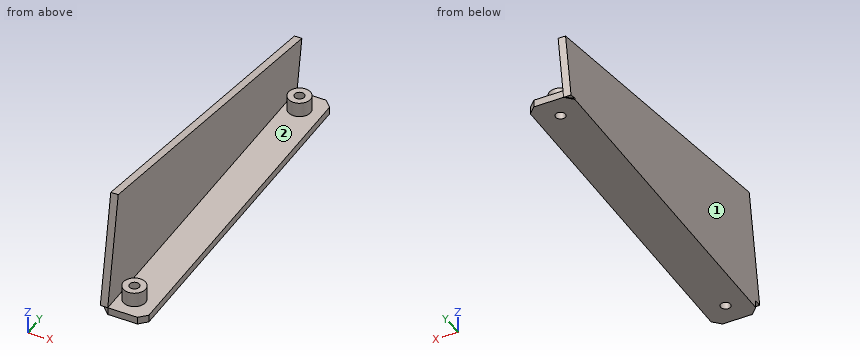
from build123d import *

# Parameters (mm, degrees)
SKETCH1_W                       = 9.525
SKETCH1_H                       = 76.2
BOSS_EXTRUDE1_DEPTH             = 1.5875
CHAMFER2_SIZE                   = 1.5875
F_97_0_0825_DIAMETER_HOLE1_D    = 2.0955
SKETCH5_R                       = 2.38125
SKETCH5_R_2                     = 1.04775
BOSS_EXTRUDE2_DEPTH             = 3.175
BOSS_EXTRUDE4_REACH             = 77.644
SKETCH7_W                       = 1.5875
SKETCH7_H                       = 75.318017262
BOSS_EXTRUDE4_DIRECTION_2_DEPTH = 12.7
BOSS_EXTRUDE5_REACH             = 79.8


with BuildPart() as part:
    # Sketch1 → Boss-Extrude1 (new body)
    with BuildSketch(Plane.XY):
        with Locations((-4.7625, 38.1)):
            Rectangle(SKETCH1_W, SKETCH1_H)
    extrude(amount=BOSS_EXTRUDE1_DEPTH)

    # Chamfer2
    chamfer2_edges = [part.edges().sort_by_distance(p)[0] for p in [
        (0, 0, 0.79375),
        (-9.525, 0, 0.79375),
        (-9.525, 76.2, 0.79375),
        (0, 76.2, 0.79375),
    ]]
    chamfer(chamfer2_edges, length=CHAMFER2_SIZE)

    # 97 _0.0825_ Diameter Hole1 (through all)
    with Locations(Plane.XY.offset(1.5875)):
        with Locations((-4.7625, 4.7625), (-4.7625, 71.4375)):
            Hole(F_97_0_0825_DIAMETER_HOLE1_D / 2)

    # Sketch5 → Boss-Extrude2 (add)
    # profile 1 of 2: a face of its own
    with BuildSketch(Plane.XY.offset(1.5875)):
        with Locations((-4.7625, 4.7625)):
            Circle(SKETCH5_R)
        with Locations((-4.7625, 4.7625)):
            Circle(SKETCH5_R_2, mode=Mode.SUBTRACT)
    # profile 2 of 2: a face of its own
    with BuildSketch(Plane.XY.offset(1.5875)):
        with Locations(Location((-4.7625, 71.4375, 0), (0, 0, 180))):
            Circle(SKETCH5_R)
        with Locations((-4.7625, 71.4375)):
            Circle(SKETCH5_R_2, mode=Mode.SUBTRACT)
    extrude(amount=BOSS_EXTRUDE2_DEPTH)

    # Boss-Extrude4: up to this face of the body (flat: up to its plane)
    boss_extrude4_end = Plane(part.part.faces().sort_by_distance((-4.7625, 38.1, 1.5875))[0])
    # Sketch7 → Boss-Extrude4 (add, up to the picked face)
    with BuildSketch(Plane(origin=(0, 2.297711148, 13.030967461), x_dir=(-1, 0, 0), z_dir=(0, -0.1736481776669307, -0.984807753012208)), mode=Mode.PRIVATE) as boss_extrude4_sk1:
        with Locations((8.73125, 37.383342149)):
            Rectangle(SKETCH7_W, SKETCH7_H)
    boss_extrude4_tool1 = split(extrude(boss_extrude4_sk1.sketch, amount=BOSS_EXTRUDE4_REACH, mode=Mode.PRIVATE), bisect_by=boss_extrude4_end, keep=Keep.BOTH, mode=Mode.PRIVATE)
    add(boss_extrude4_tool1.solids().sort_by(Axis((-8.73125, 39.113116, 6.539418), (0, -0.1736481776669307, -0.984807753012208)))[0])

    # Sketch7 → Boss-Extrude4 direction 2 (add)
    with BuildSketch(Plane(origin=(0, 2.297711148, 13.030967461), x_dir=(-1, 0, 0), z_dir=(0, -0.1736481776669307, -0.984807753012208))):
        with Locations((8.73125, 37.383342149)):
            Rectangle(SKETCH7_W, SKETCH7_H)
    extrude(amount=-BOSS_EXTRUDE4_DIRECTION_2_DEPTH)

    # Boss-Extrude5: up to this face of the body (flat: up to its plane)
    boss_extrude5_end = Plane(part.part.faces().sort_by_distance((-4.7625, 38.1, 0))[0])
    # Sketch8 → Boss-Extrude5 (add, up to the picked face)
    with BuildSketch(Plane(origin=(0, 2.297711148, 13.030967461), x_dir=(-1, 0, 0), z_dir=(0, -0.17364817766693066, -0.9848077530122081)), mode=Mode.PRIVATE) as boss_extrude5_sk1:
        Polygon((9.525, 74.993743341), (9.525, 75.04235078), (7.9375, 75.04235078), align=None)
    boss_extrude5_tool1 = split(extrude(boss_extrude5_sk1.sketch, amount=BOSS_EXTRUDE5_REACH, mode=Mode.PRIVATE), bisect_by=boss_extrude5_end, keep=Keep.BOTH, mode=Mode.PRIVATE)
    add(boss_extrude5_tool1.solids().sort_by(Axis((-8.995833, 76.184044, 0.002814), (0, -0.17364817766693066, -0.9848077530122081)))[0])


solid = part.part
Work out the finished part from the listing and answer in its coordinate system (mm). Face numbers are marked on the shaded views. Round coordinates to 2 decimals unless told otherwise and drop trailing zeros. Write each loop counter-clockwise with the first axis right and the second up, starting at its lowest first coordinate (ties: lowest second). Pieces come first, ordered by that corner, then holes. Notation, with made-up numbers: (78.5, 87.5) - (100.5, 87.5) arc R28 ccw to (100.5, 105.5) - close; hole circle Ø1 at (-13.75, -2). An arc over 180 degrees is marked (long way). Answer in a Markdown table with one row per item. Add a question column.
1. Given pin 1 (2 mm diameter, centred on x = -1, y = 21, fed in from +Z); pin 2 (4 mm diameter, centred on x = -4, y = 70.5, fed in from +Z); pin 3 (2 mm diameter, centred on x = -8, z = 12, fed in from -Y), each flat-ended and moving along its own axis, determine where each tip first touches the part or whether it passes through.
2. Find the intervals of material crossed by line 1 along X through (y, z) = (38.5, 4.5) (1 decimal); line 2 along Z through (x, y) = (-7.5, 74); line 3 along Y through (x, z) = (-3.25, 2.75), in increasing order. Write a range as from..to.
3. The mould has two halves that part along Y. Classify the marked faces 1 and 2: +Y half, -Y half, draft (parallel to the pull), parting line (faces both ways), or undercut.
4. A cutting plane is placed at B-B, the plane y = 55.5. Determine the outline of the cut face in (x, z) (1 decimal), and give its area (3 significant figures).
5. A cutting plane is placed at A-A, the plane x = -4.5. Determine the outline of the cut face in (y, z).
6. A cutting plane is placed at D-D, the plane y = 8. Determine the outline of the cut face in (x, z) (1 decimal), and give its area (3 significant figures).
7. A cutting plane is placed at C-C, the plane z = 22. Determine the outline of the cut face in (x, y) (1 decimal), and give its area (3 significant figures).
Worked out:
| question | item | result |
|---|---|---|
| 1 | pin 1 | z = 1.59 |
| 1 | pin 2 | z = 4.76 |
| 1 | pin 3 | y = 1.66 |
| 2 | line 1 | -9.5..-7.9 |
| 2 | line 2 | 0..1.59 |
| 2 | line 3 | 2.92..6.6, 69.6..73.28 |
| 3 | face 1 | draft |
| 3 | face 2 | undercut |
| 4 | outline | (-9.5, 0) - (0, 0) - (0, 1.6) - (-7.9, 1.6) - (-7.9, 16.5) - (-9.5, 16.5) - close |
| 4 | area | 38.9 mm^2 |
| 5 | outline | (0, 0) - (3.75, 0) - (3.75, 4.76) - (2.4, 4.76) - (2.4, 1.59) - (0, 1.59) - close; (5.78, 0) - (70.42, 0) - (70.42, 4.76) - (69.07, 4.76) - (69.07, 1.59) - (7.13, 1.59) - (7.13, 4.76) - (5.78, 4.76) - close; (72.45, 0) - (76.2, 0) - (76.2, 1.59) - (73.8, 1.59) - (73.8, 4.76) - (72.45, 4.76) - close |
| 6 | outline | (-9.5, 0) - (0, 0) - (0, 1.6) - (-7.9, 1.6) - (-7.9, 24.9) - (-9.5, 24.9) - close |
| 6 | area | 52.2 mm^2 |
| 7 | outline | (-9.5, 3.6) - (-7.9, 3.6) - (-7.9, 24.6) - (-9.5, 24.6) - close |
| 7 | area | 33.3 mm^2 |
